Part model, mm, in its own coordinate system. A direction names the side the tool comes from. Round coordinates to 2 decimals unless told otherwise and drop trailing zeros. Write each loop counter-clockwise with the first axis right and the second up, starting at its lowest first coordinate (ties: lowest second). Pieces come first, ordered by that corner, then holes.
```python
from build123d import *

# Parameters (mm, degrees)
F0_R     = 3
F0_R_2   = 12
F1_DEPTH = 6
F2_R     = 15
F2_R_2   = 12
F5_R     = 3
F5_R_2   = 12
F6_DEPTH = 6


with BuildPart() as f1:
    # F0 (on Top) → F1 (new body)
    with BuildSketch(Plane.XY):
        with BuildLine():
            Line((-14, -21), (14, -21))
            ThreePointArc((14, -21), (18.9497474683, -18.9497474683), (21, -14))
            Line((21, -14), (21, 14))
            ThreePointArc((21, 14), (18.9497474683, 18.9497474683), (14, 21))
            Line((14, 21), (-14, 21))
            ThreePointArc((-14, 21), (-18.9497474683, 18.9497474683), (-21, 14))
            Line((-21, 14), (-21, -14))
            ThreePointArc((-21, -14), (-18.9497474683, -18.9497474683), (-14, -21))
        make_face()
        with Locations((-14, -14)):
            Circle(F0_R, mode=Mode.SUBTRACT)
        with Locations((14, -14)):
            Circle(F0_R, mode=Mode.SUBTRACT)
        with Locations((-14, 14)):
            Circle(F0_R, mode=Mode.SUBTRACT)
        Circle(F0_R_2, mode=Mode.SUBTRACT)
        with Locations((14, 14)):
            Circle(F0_R, mode=Mode.SUBTRACT)
    extrude(amount=F1_DEPTH)

    # F4: sweep along a path in F3
    with BuildLine(Plane.YZ) as f4_path:
        Line((0, 6), (0, 36))
        ThreePointArc((0, 36), (3.8507080753, 50.7042351666), (14.4143021224, 61.6336891935))
        Line((14.4143021224, 61.6336891935), (40.0479913159, 77.2193870711))
    # F2 (on face) → F4 (sweep)
    with BuildSketch(Plane.XY.offset(6)):
        Circle(F2_R)
        Circle(F2_R_2, mode=Mode.SUBTRACT)
    sweep(path=f4_path.line)

    # F5 (on face) → F6 (join)
    with BuildSketch(Plane(origin=(0, 63.5173139927, 38.6195548528), x_dir=(-1, 0, 0), z_dir=(0, 0.8544563064, 0.5195232626))):
        with BuildLine():
            Line((-14, 24.1747291546), (14, 24.1747291546))
            ThreePointArc((14, 24.1747291546), (18.9497474683, 26.2249816863), (21, 31.1747291546))
            Line((21, 31.1747291546), (21, 59.1747291546))
            ThreePointArc((21, 59.1747291546), (18.9497474683, 64.1244766229), (14, 66.1747291546))
            Line((14, 66.1747291546), (-14, 66.1747291546))
            ThreePointArc((-14, 66.1747291546), (-18.9497474683, 64.1244766229), (-21, 59.1747291546))
            Line((-21, 59.1747291546), (-21, 31.1747291546))
            ThreePointArc((-21, 31.1747291546), (-18.9497474683, 26.2249816863), (-14, 24.1747291546))
        make_face()
        with Locations((-14, 31.1747291546)):
            Circle(F5_R, mode=Mode.SUBTRACT)
        with Locations((14, 31.1747291546)):
            Circle(F5_R, mode=Mode.SUBTRACT)
        with Locations((0, 45.1747291546)):
            Circle(F5_R_2, mode=Mode.SUBTRACT)
        with Locations((-14, 59.1747291546)):
            Circle(F5_R, mode=Mode.SUBTRACT)
        with Locations((14, 59.1747291546)):
            Circle(F5_R, mode=Mode.SUBTRACT)
    extrude(amount=F6_DEPTH)


solid = f1.part
```
Q1. Which spindle directions (+Z, -Z, +X, -X, +Y, -Y) get a long thin tool onto all of the face, cutting with end or side? Do faces 4 (the flat face through (-0.196, 31.665, 96.7)), 5 (the cylindrical face through (11.6, 12.2, 3)), 6 (the flat face through (0, 21, 3)). Say none if no direction does.
Values follow:
face 4: +Z, +X, -X, -Y
face 5: -Z
face 6: -Z, +X, -X, +Y
Q2. Drop flat-ended pins along their axis: pin 1 (3 mm diameter, centred on x = -15.5, y = 19, fed in from -Z); pin 2 (9.5 mm diameter, centred on x = 14, y = -14, fed in from +Z); pin 3 (3 mm diameter, centred on x = 2.5, z = 4, fed in from +Y); pin 4 (8 mm diameter, centred on x = 2.5, y = 4, fed in from +Z). Give the stop position or say it passes through.
Values follow:
pin 1: stops at z = 0
pin 2: stops at z = 6
pin 3: stops at y = 21
pin 4: stops at z = 75.13
Q3. Mould opens along Z. For faces 1 (the cylindrical face through (-14.985, 0.66, 21.21)), 2 (the cylindrical face through (19, 18.9, 3)), 3 (the cylindrical face through (18.9, 32.7, 94.99)) say: +Z half, -Z half, draft (parallel to the pull), parting line (faces both ways), or undercut.
Values follow:
face 1: undercut
face 2: draft
face 3: +Z half
Q4. Cut at A-A on x = -4.5. Write the cut outline in (y, z), plus the area to 3 significant figures.
Values follow:
outline: (-21, 0) - (-11.12, 0) - (-11.12, 36) arc R41.12 cw to (8.63, 71.14) - (39.4, 89.84) - (34.26, 98.28) - (29.14, 95.16) - (32.61, 89.45) - (6.98, 73.86) arc R44.31 ccw to (-14.31, 36) - (-14.31, 6) - (-21, 6) - close; (11.12, 0) - (21, 0) - (21, 6) - (14.31, 6) - (14.31, 36) arc R15.69 cw to (21.85, 49.41) - (47.48, 64.99) - (50.96, 59.28) - (56.08, 62.39) - (50.95, 70.83) - (20.19, 52.13) arc R18.88 ccw to (11.12, 36) - close
area: 815 mm2
Q5. Cut at B-B on x = 3. Write the cut outline in (y, z).
Values follow:
outline: (-21, 0) - (-11.62, 0) - (-11.62, 36) arc R41.62 cw to (8.38, 71.56) - (39.14, 90.26) - (34.26, 98.28) - (29.14, 95.16) - (32.41, 89.78) - (6.78, 74.19) arc R44.7 ccw to (-14.7, 36) - (-14.7, 6) - (-21, 6) - close; (11.62, 0) - (21, 0) - (21, 6) - (14.7, 6) - (14.7, 36) arc R15.3 cw to (22.05, 49.08) - (47.68, 64.66) - (50.96, 59.28) - (56.08, 62.39) - (51.21, 70.41) - (20.45, 51.71) arc R18.38 ccw to (11.62, 36) - close
Q6. Wall check: L1, parallel to Y at x = 14, z = 4.2; L2, parallel to Z at x = 7, y = 31.5; L3, parallel to Y at x = 0, z = 11. Give the ranges that are in metal, low to high.
Values follow:
L1: y = -21 to -17, -11 to 11, 17 to 21
L2: z = 56.5 to 60.62, 83.43 to 87.55, 91.28 to 96.6
L3: y = -15 to -12, 12 to 15
